Could you check a few things on this model? Use its own coordinates, in mm. Face numbers are marked on the shaded views. A direction names the side the tool comes from. Coordinates: 2 decimals unless noted, no trailing zeros. Loops run counter-clockwise (first coordinate to the right, second up) from the corner with the lowest first, then second, coordinate; pieces in that order, holes last. Notation, with made-up numbers: (55.25, 47) -> (75.25, 47) arc R20 ccw to (75.25, 68) -> close; hole circle Ø5 at (-6.75, -4.75). An arc over 180 degrees is marked (long way). One line per question, with ' | ' between items. Start each with the question number.
(1) I'm going to push flat-ended pins straight in: pin 1 Ø1.5 at (x, z) = (1.5, 26) entering from -Y; pin 2 Ø2 at (x, y) = (0, 0) entering from +Z; pin 3 Ø1.5 at (x, y) = (4.5, -1.5) entering from +Z. Where does each tip first touch, or does it pass through?
(2) If we mould it in two halves opening along X, with no side actions, what happens to the marked faces 1, 2 and 3? For each: pulls with the +X half, pulls with the -X half, needs draft (parallel to the pull), parting line crosses it, or undercut.
(3) Which directions (+Z, -Z, +X, -X, +Y, -Y) give clear straight access to the entire face, cutting with the end or side of a thin tool? Please do the marked faces 4 and 5.
(4) Suppose I cut it at A-A (z = -5). Please give me the cut outline in (x, y).
(5) Suppose I cut it at C-C (z = 20). Please give me the cut outline in (x, y), plus the area to 3 significant figures.
(6) Suppose I cut it at B-B (x = -4.5). Please give me the cut outline in (y, z), plus the area to 3 significant figures.
(7) If I drill on line 1 along Y through (x, z) = (0, 30.5); line 2 along Z through (x, y) = (-5, 0.5); line 3 along Y through (x, z) = (-2.75, 14), over which ranges is the centre line in solid material (lowest first)?
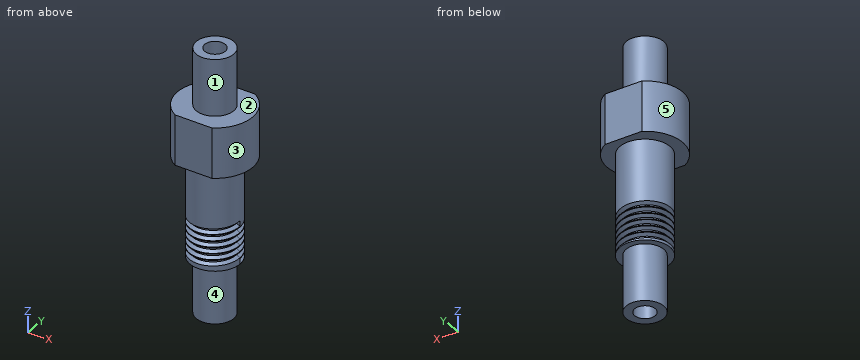
```python
from build123d import *

# Parameters (mm, degrees)
SKETCH1_R                 = 4
BOSS_EXTRUDE1_DEPTH       = 16
SKETCH2_R                 = 6
BOSS_EXTRUDE2_DEPTH       = 8
SKETCH3_R                 = 3
BOSS_EXTRUDE3_DEPTH       = 9
BOSS_EXTRUDE4_START       = 9
SKETCH8_R                 = 3
BOSS_EXTRUDE4_DEPTH       = 9
M4X0_7_TAPPED_HOLE2_D     = 3.3
M4X0_7_TAPPED_HOLE2_DEPTH = 10
M4X0_7_TAPPED_HOLE2_TIP   = 0.991420021
THREAD1_PITCH             = 1
M4X0_7_TAPPED_HOLE3_D     = 3.3
M4X0_7_TAPPED_HOLE3_DEPTH = 10
M4X0_7_TAPPED_HOLE3_TIP   = 0.991420021
CUT_EXTRUDE1_START        = -10
CUT_EXTRUDE1_DEPTH        = 10


with BuildPart() as part:
    # Sketch1 → Boss-Extrude1 (new body)
    with BuildSketch(Plane.XY):
        Circle(SKETCH1_R)
    extrude(amount=BOSS_EXTRUDE1_DEPTH)

    # Sketch2 → Boss-Extrude2 (add)
    with BuildSketch(Plane.XY.offset(16)):
        Circle(SKETCH2_R)
    extrude(amount=BOSS_EXTRUDE2_DEPTH)

    # Sketch3 → Boss-Extrude3 (add)
    with BuildSketch(Plane(origin=(0, 0, 0), x_dir=(-1, 0, 0), z_dir=(0, 0, -1))):
        Circle(SKETCH3_R)
    extrude(amount=BOSS_EXTRUDE3_DEPTH)

    # Sketch8 → Boss-Extrude4 (add)
    with BuildSketch(Plane.XY.offset(24).offset(BOSS_EXTRUDE4_START)):
        with Locations(Location((0, 0, 0), (0, 0, 180))):
            Circle(SKETCH8_R)
    extrude(amount=-BOSS_EXTRUDE4_DEPTH)

    # M4x0.7 Tapped Hole2
    with Locations(Plane.XY.offset(33)):
        with Locations((0, 0)):
            Hole(M4X0_7_TAPPED_HOLE2_D / 2, depth=M4X0_7_TAPPED_HOLE2_DEPTH)
            with Locations((0, 0, -(M4X0_7_TAPPED_HOLE2_DEPTH + M4X0_7_TAPPED_HOLE2_TIP / 2))):  # 118° drill point
                Cone(0, M4X0_7_TAPPED_HOLE2_D / 2, M4X0_7_TAPPED_HOLE2_TIP, mode=Mode.SUBTRACT)

    # Thread1: the profile of Thread Profile2 profile screwed along a right-hand helix of 6 turns, 8 arcs to a turn; built about Z, then put on its axis
    thread1_z = Axis((0, 0, 0), (0, 0, 1))
    thread1_corners = [(4.0003, 0, -0.000173205), (4.0003, 0, 0.875173202), (3.458734125, 0, 0.562499999), (3.458734125, 0, 0.312499999)]
    with BuildLine(mode=Mode.PRIVATE) as thread1_profile:
        Line(thread1_corners[0], thread1_corners[1])
        Line(thread1_corners[1], thread1_corners[2])
        Line(thread1_corners[2], thread1_corners[3])
        Line(thread1_corners[3], thread1_corners[0])
    thread1_cap = Face(thread1_profile.wire())
    thread1_turn_angles = [0, 22.5, 45, 67.5, 90, 112.5, 135, 157.5, 180, 202.5, 225, 247.5, 270, 292.5, 315, 337.5, 360]
    thread1_turn_weights = [1, 0.9238795325112867, 1, 0.9238795325112867, 1, 0.9238795325112867, 1, 0.9238795325112867, 1, 0.9238795325112867, 1, 0.9238795325112867, 1, 0.9238795325112867, 1, 0.9238795325112867, 1]
    thread1_turn_rails = [Edge.make_bspline([Vector(p[0], p[1], 0).rotate(thread1_z, thread1_turn_angles[k]) / thread1_turn_weights[k] + Vector(0, 0, p[2] + THREAD1_PITCH * thread1_turn_angles[k] / 360) for k in range(17)], [0, 0, 0, 1, 1, 2, 2, 3, 3, 4, 4, 5, 5, 6, 6, 7, 7, 8, 8, 8], 2, thread1_turn_weights) for p in thread1_corners]
    thread1_turn_sides = [Face.make_surface_from_curves(thread1_turn_rails[p[0]], thread1_turn_rails[p[1]]) for p in [(0, 1), (1, 2), (2, 3), (3, 0)]]
    thread1 = Plane(origin=(0, 0, 0), x_dir=(1, 0, 0), z_dir=(0, 0, 1)) * Solid(Shell([*[p.moved(Location((0, 0, THREAD1_PITCH * i))) for i in range(6) for p in thread1_turn_sides], thread1_cap, thread1_cap.rotate(thread1_z, 2160).moved(Location((0, 0, THREAD1_PITCH * 2160 / 360)))]))
    add(thread1, mode=Mode.SUBTRACT)

    # M4x0.7 Tapped Hole3
    with Locations(Plane(origin=(0, 0, -9), x_dir=(-1, 0, 0), z_dir=(0, 0, -1))):
        with Locations((0, 0)):
            Hole(M4X0_7_TAPPED_HOLE3_D / 2, depth=M4X0_7_TAPPED_HOLE3_DEPTH)
            with Locations((0, 0, -(M4X0_7_TAPPED_HOLE3_DEPTH + M4X0_7_TAPPED_HOLE3_TIP / 2))):  # 118° drill point
                Cone(0, M4X0_7_TAPPED_HOLE3_D / 2, M4X0_7_TAPPED_HOLE3_TIP, mode=Mode.SUBTRACT)

    # Sketch36 → Cut-Extrude1 (cut)
    with BuildSketch(Plane.XY.offset(24).offset(CUT_EXTRUDE1_START)):
        with BuildLine():
            Line((-2.90430853, 5.250237325), (3.094684634, 5.140323629))
            ThreePointArc((3.094684634, 5.140323629), (0.109913695, 5.998993164), (-2.90430853, 5.250237325))
        make_face()
        with BuildLine():
            ThreePointArc((-3.094684634, -5.140323629), (-0.109913695, -5.998993164), (2.90430853, -5.250237325))
            Line((2.90430853, -5.250237325), (-3.094684634, -5.140323629))
        make_face()
    extrude(amount=CUT_EXTRUDE1_DEPTH, mode=Mode.SUBTRACT)


solid = part.part
```
Checks:
1) pin 1: stops at y = -2.9 | pin 2: stops at z = 22.61 | pin 3: stops at z = 24
2) face 1: parting line crosses it | face 2: needs draft | face 3: pulls with the +X half
3) face 4: -Z | face 5: +Z, -Z, -X
4) outline: circle Ø6 at (0, 0); hole circle Ø3.3 at (0, 0)
5) outline: (-3.09, -5.14) -> (2.9, -5.25) arc R6 ccw to (3.09, 5.14) -> (-2.9, 5.25) arc R6 ccw to start | area: 107 mm^2
6) outline: (-3.97, 16) -> (3.97, 16) -> (3.97, 24) -> (-3.97, 24) -> close | area: 63.5 mm^2
7) line 1: y = -3 to -1.65, 1.65 to 3 | line 2: z = 16 to 24 | line 3: y = -2.9 to 2.9
